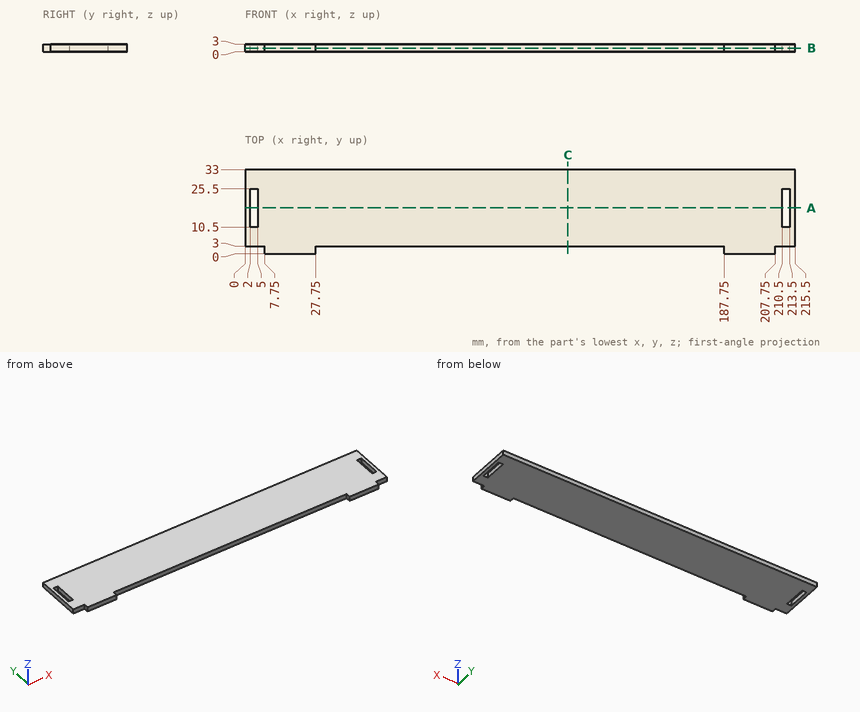
Design review of the part shown in the three views and the two pictorial views. Dimensions are in mm from the part's minimum x, y and z. Give positions to 0.01 mm unless a question says otherwise; leave off trailing zeros. Loops run counter-clockwise (first coordinate to the right, second up) from the corner with the lowest first, then second, coordinate; pieces in that order, holes last. Notation, with made-up numbers: (76.25, 27.5) - (109.25, 27.5) arc R17 cw to (109.25, 36.5) - close; hole circle Ø9 at (62, 0.5). An arc over 180 degrees is marked (long way). Answer as a JSON object with one key per item and string values.
Q1. Add section A-A on y = 18. State the section outline as (x, z) points.
Worked out:
{"outline": "(0, 0) - (2, 0) - (2, 3) - (0, 3) - close; (5, 0) - (210.5, 0) - (210.5, 3) - (5, 3) - close; (213.5, 0) - (215.5, 0) - (215.5, 3) - (213.5, 3) - close"}
Q2. To check wall thickness, follow line 1 along X through (y, z) = (13, 2.65); line 2 along X through (y, z) = (2, 2); line 3 along Y through (x, z) = (185.5, 1.2). State the ranges of each line that lie inside material, in increasing order.
Worked out:
{"line 1": "x = 0 to 2, 5 to 210.5, 213.5 to 215.5", "line 2": "x = 7.75 to 27.75, 187.75 to 207.75", "line 3": "y = 3 to 33"}
Q3. Add section C-C on x = 126.5. State the section outline as (y, z) points, plus the area to 3 significant figures.
Worked out:
{"outline": "(3, 0) - (33, 0) - (33, 3) - (3, 3) - close", "area": "90.0 mm^2"}
Q4. Insertion check: pin 1 (1.5 mm diameter, centred on y = 1.5, z = 2, fed in from +X); pin 2 (0.9 mm diameter, centred on x = 210.5, z = 1, fed in from -Y). Each pin has a flat end and moves straight along its axis. Give the tip position at first contact, or say it passes through.
Worked out:
{"pin 1": "stops at x = 207.75", "pin 2": "stops at y = 3"}
Q5. Add section B-B on z = 1.4. State the section outline as (x, y) points, plus the area to 4 significant figures.
Worked out:
{"outline": "(0, 3) - (7.75, 3) - (7.75, 0) - (27.75, 0) - (27.75, 3) - (187.75, 3) - (187.75, 0) - (207.75, 0) - (207.75, 3) - (215.5, 3) - (215.5, 33) - (0, 33) - close; hole (2, 10.5) - (5, 10.5) - (5, 25.5) - (2, 25.5) - close; hole (210.5, 10.5) - (213.5, 10.5) - (213.5, 25.5) - (210.5, 25.5) - close", "area": "6,495 mm^2"}
